Geometry check sheet. Reference: drawing and pictorial views, mm from the part's lowest x, y, z. A direction names the side the tool comes from. Give positions to 0.01 mm unless a question says otherwise; leave off trailing zeros. Write each loop counter-clockwise with the first axis right and the second up, starting at its lowest first coordinate (ties: lowest second). Pieces come first, ordered by that corner, then holes. Notation, with made-up numbers: (1, 55.5) -> (16, 55.5) arc R22 ccw to (16, 65.5) -> close; hole circle Ø9 at (45.25, 80). An arc over 180 degrees is marked (long way). Answer as CSV lines item,"result".
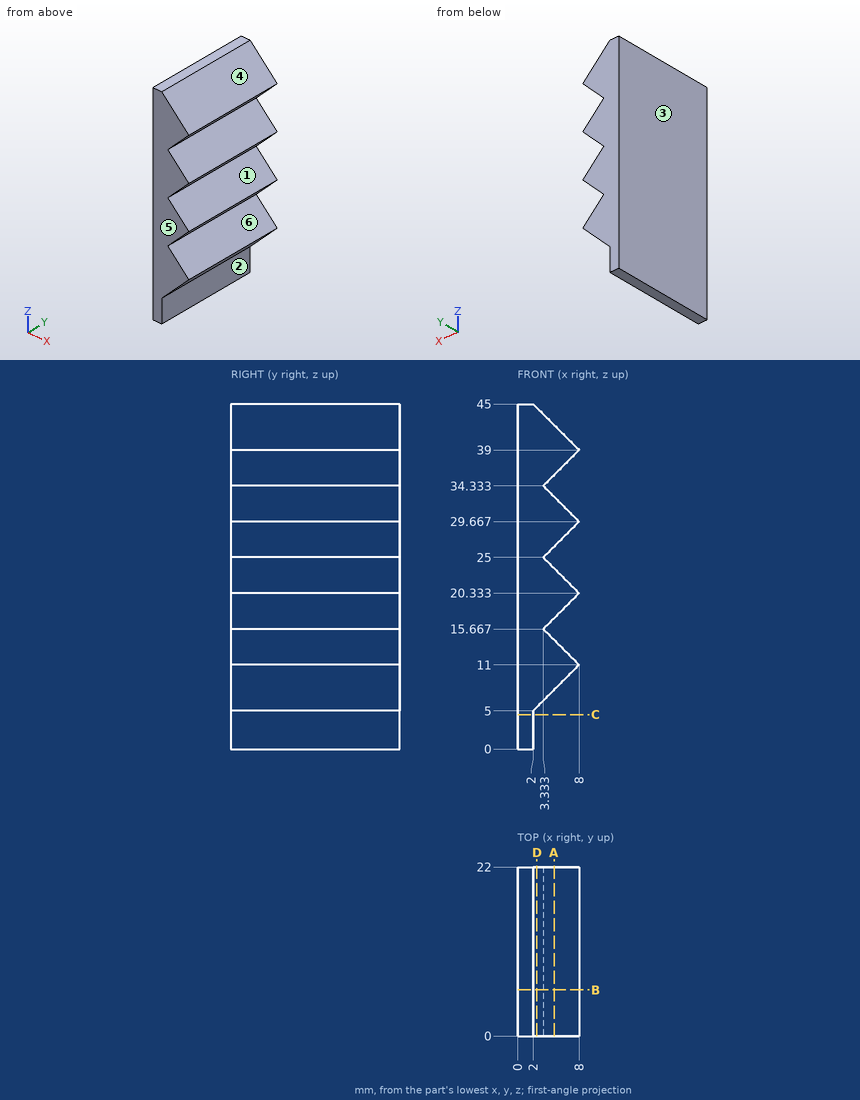
1) Tool access check on the marked faces 1, 2 and 3. Record the directions out of +Z, -Z, +X, -X, +Y, -Y that give a thin tool (end or side, any length) a straight path to the whole face; none if there is none.
Reported:
face 1,"+X, +Y, -Y"
face 2,"-Z, +X, +Y, -Y"
face 3,"+Z, -Z, -X, +Y, -Y"
2) Scan lines: line 1 along Z through (x, y) = (7, 20.75) (1 decimal); line 2 along X through (y, z) = (8, 8); line 3 along Z through (x, y) = (4.5, 8.25) (1 decimal). Record each from-to range of solid material in increasing order.
Reported:
line 1,"10 to 12, 19.3 to 21.3, 28.7 to 30.7, 38 to 40"
line 2,"0 to 5"
line 3,"7.5 to 14.5, 16.8 to 23.8, 26.2 to 33.2, 35.5 to 42.5"
3) Section check C-C (z = 4.5). Record the boundary of the cut face in (x, y), and give its area (3 significant figures).
Reported:
outline,"(0, 0) -> (2, 0) -> (2, 22) -> (0, 22) -> close"
area,"44.0 mm²"
4) Depth check by flat-ended pin: pin 1 (5 mm diameter, centred on y = 2, z = 35, fed in from +X); pin 2 (2 mm diameter, centred on x = 3.5, y = 17.5, fed in from +Z); pin 3 (4 mm diameter, centred on y = 16, z = 16.5, fed in from +X). Enter the tip coordinate at first touch or a pass-through.
Reported:
pin 1,"x = 6.5"
pin 2,"z = 44.5"
pin 3,"x = 6.17"
5) Draft check along Z on the marked faces 4, 5 and 6. Enter one of: +Z half, -Z half, draft (parallel to the pull), parting line (faces both ways), or undercut.
Reported:
face 4,"+Z half"
face 5,"draft"
face 6,"undercut"
6) Section check B-B (y = 6). Record the boundary of the cut face in (x, z), and give its area (3 significant figures).
Reported:
outline,"(0, 0) -> (2, 0) -> (2, 5) -> (8, 11) -> (3.33, 15.67) -> (8, 20.33) -> (3.33, 25) -> (8, 29.67) -> (3.33, 34.33) -> (8, 39) -> (2, 45) -> (0, 45) -> close"
area,"229 mm²"
7) Section check A-A (x = 4.75). Record the boundary of the cut face in (y, z).
Reported:
outline,"(0, 7.75) -> (22, 7.75) -> (22, 14.25) -> (0, 14.25) -> close; (0, 17.08) -> (22, 17.08) -> (22, 23.58) -> (0, 23.58) -> close; (0, 26.42) -> (22, 26.42) -> (22, 32.92) -> (0, 32.92) -> close; (0, 35.75) -> (22, 35.75) -> (22, 42.25) -> (0, 42.25) -> close"
8) Section check D-D (x = 2.5). Record the boundary of the cut face in (y, z), and give its area (3 significant figures).
Reported:
outline,"(0, 5.5) -> (22, 5.5) -> (22, 44.5) -> (0, 44.5) -> close"
area,"858 mm²"
